Design review of the part shown in the three views and the two pictorial views. Dimensions are in mm from the part's minimum x, y and z. Give positions to 0.01 mm unless a question says otherwise; leave off trailing zeros. Loops run counter-clockwise (first coordinate to the right, second up) from the corner with the lowest first, then second, coordinate; pieces in that order, holes last. Notation, with made-up numbers: M 56,-19.5 L 115,-19.5 A14 ccw 115,-14.5 Z; hole C 74.5,56.25 d6. An arc over 180 degrees is marked long. Return JSON: item names as keys, results as strings. Group by question number.
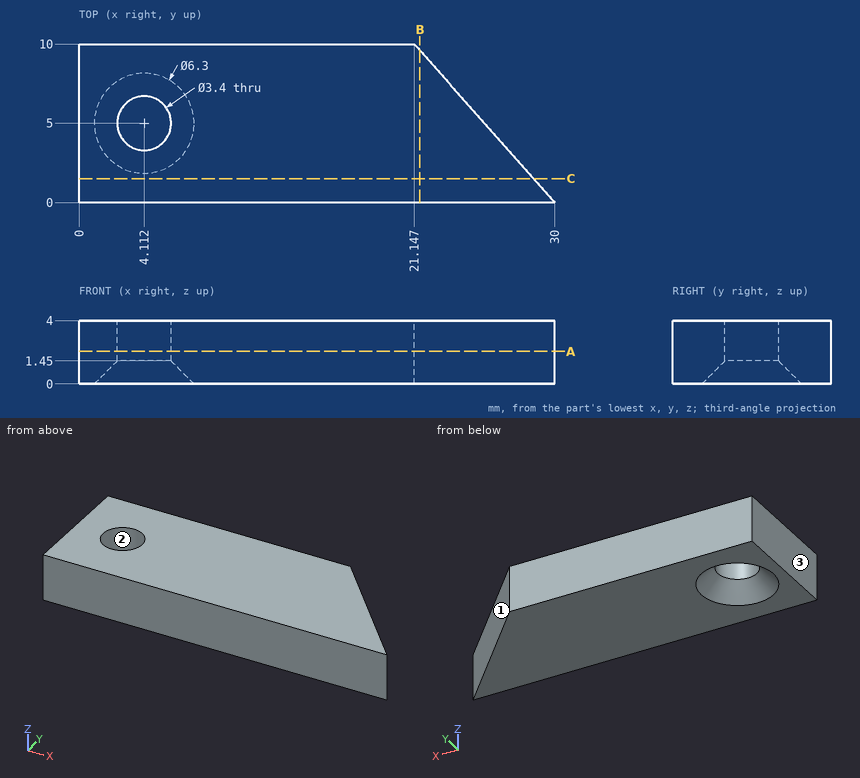
(1) Add section B-B (x = 21.5). Write out the cut boundary in (y, z), and give its area (3 significant figures).
(2) For pin 1 (1 mm diameter, centred on y = 8.5, z = 1, fed in from +X); pin 2 (3 mm diameter, centred on x = 4.11, y = 5, fed in from -Z); pin 3 (2 mm diameter, centred on y = 2.5, z = 3, fed in from +X), all flat-tipped, find the tip position at first contact; note any pin that passes through.
(3) Mouldability with a two-part tool opening along Y and no side actions: class the marked faces 1, 2 and 3 as released by +Y, released by -Y, zero draft, split by the parting line, or undercut.
(4) For probe 1 along X at (y, z) = (5, 3.4) (1 decimal); probe 2 along X at (y, z) = (6.5, 3) (1 decimal); probe 3 along Z at (x, y) = (3.75, 7.5) (1 decimal), list the stretches that pass through material, from the lowest coordinate up.
(5) Add section C-C (y = 1.5). Write out the cut boundary in (x, z).
(6) Add section A-A (z = 2.05). Write out the cut boundary in (x, y).
Verdict:
{
 "1": {"outline": "M 0,0 L 9.6,0 L 9.6,4 L 0,4 Z", "area": "38.4 mm²"},
 "2": {"pin 1": "stops at x = 22.92", "pin 2": "passes through", "pin 3": "stops at x = 28.67"},
 "3": {"face 1": "released by +Y", "face 2": "undercut", "face 3": "zero draft"},
 "4": {"probe 1": "x = 0 to 2.4, 5.8 to 25.6", "probe 2": "x = 0 to 3.3, 4.9 to 24.2", "probe 3": "z = 0.6 to 4"},
 "5": {"outline": "M 0,0 L 28.67,0 L 28.67,4 L 0,4 Z"},
 "6": {"outline": "M 0,0 L 30,0 L 21.15,10 L 0,10 Z; hole C 4.11,5 d3.4"}
}
